The drawing under review shows one solid part. Ordinate dimensions are in mm from its lowest x, y, z. Coordinates: 2 decimals unless noted, no trailing zeros. Write each loop counter-clockwise with the first axis right and the second up, starting at its lowest first coordinate (ties: lowest second). Pieces come first, ordered by that corner, then holes.
Q1. Take a section at C-C (z = 3). Give the boundary of the cut face in (x, y).
Q2. For probe 1 along Y at (x, z) = (5, 6.25); probe 2 along Z at (x, y) = (7.5, 1); probe 3 along X at (y, z) = (6.5, 6.5), list the stretches that pass through material, from the lowest coordinate up.
Q3. Insertion check: pin 1 (6 mm diameter, centred on x = 5, y = 5, fed in from +Z); pin 2 (6 mm diameter, centred on y = 8, z = 6.5, fed in from +X); pin 3 (3 mm diameter, centred on y = 5, z = 3.5, fed in from -X); pin 4 (1 mm diameter, centred on y = 7, z = 3.5, fed in from +X). Each pin has a flat end and moves straight along its axis. Give the tip position at first contact, or say it passes through.
Q4. Take a section at A-A (y = 5). Give the boundary of the cut face in (x, z).
Q5. Mouldability with a two-part tool opening along Z and no side actions: class the marked faces 1, 2 and 3 as pulls with the +Z half, pulls with the -Z half, needs draft (parallel to the pull), parting line crosses it, or undercut.
Q6. Take a section at D-D (z = 11.25). Give the boundary of the cut face in (x, y).
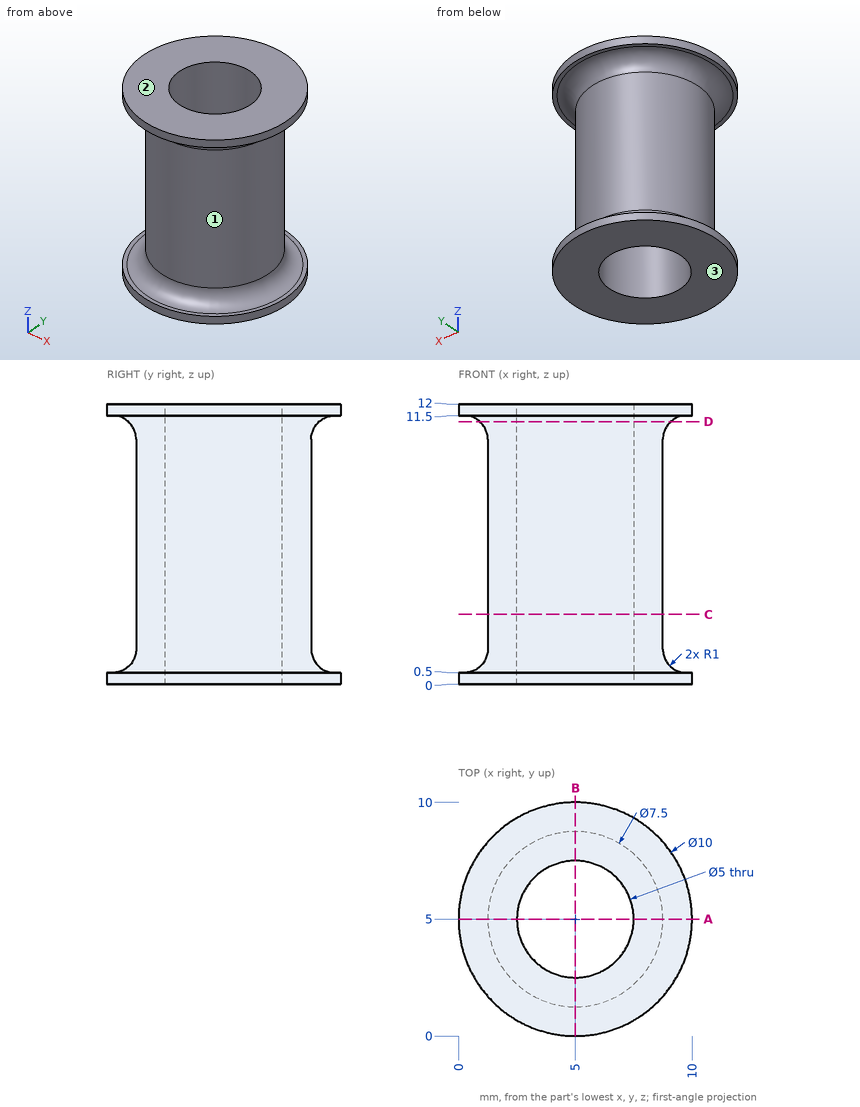
Response:
1. outline: circle Ø7.5 at (5, 5); hole circle Ø5 at (5, 5)
2. probe 1: y = 1.25 to 2.5, 7.5 to 8.75
2. probe 2: z = 0 to 0.5, 11.5 to 12
2. probe 3: x = 1.56 to 3, 7 to 8.44
3. pin 1: stops at z = 12
3. pin 2: stops at x = 8.75
3. pin 3: stops at x = 1.25
3. pin 4: stops at x = 8.44
4. outline: (0, 0) - (2.5, 0) - (2.5, 12) - (0, 12) - (0, 11.5) - (0.25, 11.5) arc R1 cw to (1.25, 10.5) - (1.25, 1.5) arc R1 cw to (0.25, 0.5) - (0, 0.5) - close; (7.5, 0) - (10, 0) - (10, 0.5) - (9.75, 0.5) arc R1 cw to (8.75, 1.5) - (8.75, 10.5) arc R1 cw to (9.75, 11.5) - (10, 11.5) - (10, 12) - (7.5, 12) - close
5. face 1: undercut
5. face 2: pulls with the +Z half
5. face 3: pulls with the -Z half
6. outline: circle Ø8.18 at (5, 5); hole circle Ø5 at (5, 5)
